Read the model definition and answer for the solid it produces. Units are mm, in the model's axes. Face numbers are marked on the shaded views. A direction names the side the tool comes from. Coordinates: 2 decimals unless noted, no trailing zeros. Loops run counter-clockwise (first coordinate to the right, second up) from the corner with the lowest first, then second, coordinate; pieces in that order, holes last. Notation, with made-up numbers: M 37,54.5 L 78,54.5 A15 ccw 78,77.5 Z; hole C -1,13.25 d8. An arc over 180 degrees is marked long. Use one line per item in the form item = value. Start each with the question number.
1. The part is cut by section A-A (y = 5.25). Give the vertices of the cut face in (x, z).
2. Find the intervals of material crossed by probe 1 along X at (y, z) = (7.75, -21.5); probe 2 along Z at (x, y) = (-28, 7.75); probe 3 along Z at (x, y) = (-74, 7), in increasing order. Write a range as [from, to].
3. A tool of negligible diameter and unlimited length cuts with its end or side. For the marked faces 1 and 2, from which of +Z, -Z, +X, -X, +Y, -Y can it reach the whole face along a straight path? Write none if from no direction.
4. The part is cut by section B-B (x = -136.5). Give the vertices of the cut face in (y, z), plus the area to 3 significant figures.
5. Flat-ended cylindrical pins translate along their axes: pin 1 (1 mm diameter, centred on y = 4, z = -21, fed in from -X); pin 2 (5 mm diameter, centred on x = -147.5, y = 5, fed in from -Z); pin 3 (4 mm diameter, centred on x = -99.5, y = 2.5, fed in from -Z); pin 4 (5 mm diameter, centred on x = -84, z = -52.5, fed in from -Y). Find the tip coordinate at first contact, or state that the pin passes through.
6. For a pull along Z with two mould halves and no side action, classify the marked faces 3, 4, 5 and 6 as released by +Z, released by -Z, zero draft, split by the parting line, or undercut.
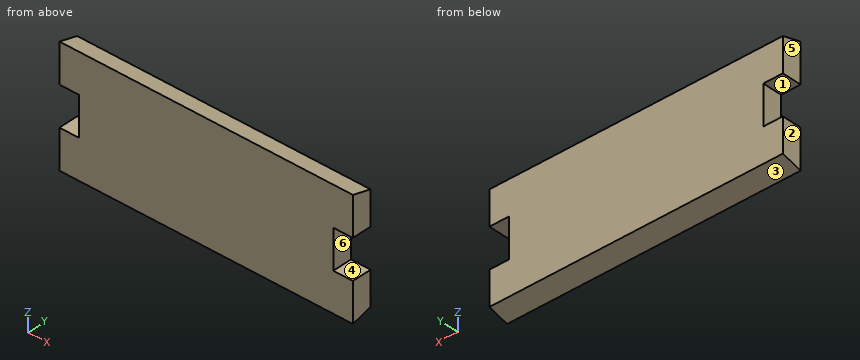
from build123d import *

# Parameters (mm, degrees)
BOSS_EXTRUDE1_DEPTH = 10
DRAFT21_ANGLE       = -15
DRAFT22_ANGLE       = -15


with BuildPart() as part:
    # Sketch1 → Boss-Extrude1 (new body)
    with BuildSketch(Plane(origin=(0, 0, 0), x_dir=(1, 0, 0), z_dir=(0, 1, 0))):
        Polygon((0, 0), (0, 20), (-10, 20), (-10, 40), (0, 40), (0, 60), (-150, 60), (-150, 40), (-140, 40), (-140, 20), (-150, 20), (-150, 0), align=None)
    extrude(amount=BOSS_EXTRUDE1_DEPTH)

    # Draft21
    draft21_faces = [part.faces().sort_by_distance(p)[0] for p in [
        (-75, 5, 0),
    ]]
    draft(draft21_faces, Plane(origin=(0, 0, 0), x_dir=(0, 0, -1), z_dir=(0, -1, 0)), DRAFT21_ANGLE)

    # Draft22
    draft22_faces = [part.faces().sort_by_distance(p)[0] for p in [
        (-75, 5, -60),
    ]]
    draft(draft22_faces, Plane(origin=(0, 0, 0), x_dir=(0, 0, -1), z_dir=(0, -1, 0)), DRAFT22_ANGLE)


solid = part.part
Computed values:
q1.outline = M -150,-58.59 L 0,-58.59 L 0,-40 L -10,-40 L -10,-20 L 0,-20 L 0,-1.41 L -150,-1.41 L -150,-20 L -140,-20 L -140,-40 L -150,-40 Z
q2.probe_1 = [-140, -10]
q2.probe_2 = [-57.92, -2.08]
q2.probe_3 = [-58.12, -1.88]
q3.face_1 = -X, +Y, -Y
q3.face_2 = +Z, -Z, -X, +Y, -Y
q4.outline = M 0,-60 L 10,-57.32 L 10,-2.68 L 0,0 Z
q4.area = 573 mm²
q5.pin_1 = -140
q5.pin_2 = -59.33
q5.pin_3 = -59.87
q5.pin_4 = 0
q6.face_3 = released by -Z
q6.face_4 = undercut
q6.face_5 = zero draft
q6.face_6 = undercut
